```python
from build123d import *

# Parameters (mm, degrees)
F0_W     = 72
F0_H     = 50
F0_R     = 3
F1_DEPTH = 5
F2_R     = 1.75
F3_DEPTH = 25
F4_R     = 1.75
F5_DEPTH = 25


with BuildPart() as f1:
    # F0 (on Front) → F1 (new body)
    with BuildSketch(Plane.XZ):
        Rectangle(F0_W, F0_H)
        with Locations((0, -2.52)):
            Circle(F0_R, mode=Mode.SUBTRACT)
    extrude(amount=F1_DEPTH)

    # F2 (on face) → F3 (cut)
    with BuildSketch(Plane(origin=(-36, 0, 0), x_dir=(0, -1, 0), z_dir=(-1, 0, 0))):
        with Locations((2.5, 22.5)):
            Circle(F2_R)
        with Locations((2.5, -22.5)):
            Circle(F2_R)
        with Locations((2.5, 0)):
            Circle(F2_R)
    extrude(amount=-F3_DEPTH, mode=Mode.SUBTRACT)

    # F4 (on face) → F5 (cut)
    with BuildSketch(Plane.YZ.offset(36)):
        with Locations((-2.5, 0)):
            Circle(F4_R)
        with Locations((-2.5, 22.5)):
            Circle(F4_R)
        with Locations((-2.5, -22.5)):
            Circle(F4_R)
    extrude(amount=-F5_DEPTH, mode=Mode.SUBTRACT)


solid = f1.part
```
Model file for the job. Use its own axes, mm. A direction names the side the tool comes from. Round coordinates to 2 decimals unless told otherwise and drop trailing zeros. Loops run counter-clockwise (first coordinate to the right, second up) from the corner with the lowest first, then second, coordinate; pieces in that order, holes last. Notation, with made-up numbers: M 33,28.25 L 60,28.25 A15 cw 60,42.25 Z; hole C 79.5,62.25 d9. An arc over 180 degrees is marked long. Put each result on its own line as item: value. Start each with the question number.
Item 1: 3-axis set-ups, long thin cutter, end or side, ignore diameter. For faces 5 (the face through (23.675, -2.728, 24.235)), 6 (the face through (-0.65, -2.46, -5.45)), 7 (the face through (-23.675, -2.272, -20.765)): which of +Z, -Z, +X, -X, +Y, -Y reach the whole face in a straight line?
Item 2: Drop flat-ended pins along their axis: P1, Ø3, axis at y = -2.5, z = 0, coming from the -X side; P2, Ø1, axis at y = -3, z = 22, coming from the +X side. Give the stop position or say it passes through.
Item 3: Drill centre lines: line 1 along Z through (x, y) = (-21.25, -2.5); line 2 along Z through (x, y) = (-19.5, -1.9); line 3 along Z through (x, y) = (0, -1.25). Where is each one in solid material? Low to high.
Item 4: Cut at D-D (x = 0). List the corners of the cut face in (y, z).
Item 5: Cut at A-A (x = -28.5). List the corners of the cut face in (y, z), then the cut area to 3 significant figures.
Item 6: Mould opens along Y. For faces 1 (the face through (23.675, -0.883, -0.67)), 2 (the face through (-1, 0, 6)), 3 (the face through (-1, -2, -25)), 4 (the face through (23.675, -2.728, -20.765)) say: released by +Y, released by -Y, zero draft, split by the parting line, or undercut.
Item 7: Cut at B-B (z = -2.52). List the corners of the cut face in (x, y), then the cut area to 3 significant figures.
Answer block:
1. face 5: +X
1. face 6: +Y, -Y
1. face 7: -X
2. P1: x = -11
2. P2: x = 11
3. line 1: -25 to -24.25, -20.75 to -1.75, 1.75 to 20.75, 24.25 to 25
3. line 2: -25 to -24.14, -20.86 to -1.64, 1.64 to 20.86, 24.14 to 25
3. line 3: -25 to -5.52, 0.48 to 25
4. outline: M -5,-25 L 0,-25 L 0,-5.52 L -5,-5.52 Z; M -5,0.48 L 0,0.48 L 0,25 L -5,25 Z
5. outline: M -5,-25 L 0,-25 L 0,25 L -5,25 Z; hole C -2.5,-22.5 d3.5; hole C -2.5,0 d3.5; hole C -2.5,22.5 d3.5
5. area: 221 mm2
6. face 1: undercut
6. face 2: released by +Y
6. face 3: zero draft
6. face 4: undercut
7. outline: M -36,-5 L -3,-5 L -3,0 L -36,0 Z; M 3,-5 L 36,-5 L 36,0 L 3,0 Z
7. area: 330 mm2
